CAD build for the part. Positions are in the model's coordinates, mm. A direction names the side the tool comes from. Round coordinates to 2 decimals unless told otherwise and drop trailing zeros. Put each result on its own line as item: value. Start each with the question number.
Item 1: Mould opens along Z. For faces 1 (the flat face through (920.75, 748, -19)), 2 (the flat face through (548, 2136.775, -466)), 3 (the flat face through (83, 1142, -3.175)) say: released by +Z, released by -Z, zero draft, split by the parting line, or undercut.
Item 2: 3-axis set-ups, long thin cutter, end or side, ignore diameter. For faces 4 (the flat face through (914.918, 1053, -454)), 5 (the flat face through (838, 1142, -917.575)), 6 (the flat face through (917.575, 1056, -454)): which of +Z, -Z, +X, -X, +Y, -Y reach the whole face in a straight line?
Item 3: Drill centre lines: line 1 (X direction, y = 477, z = -827.5) (3 decimals); line 2 (Z direction, x = 99, y = 528) (3 decimals); line 3 (Y direction, x = 826, z = -126) (3 decimals). Where is each one in solid material? Low to high. Write a range as from..to.
Item 4: Cut at B-B (z = -780.5). Count the separate pieces of the cut face and the enclosed holes in it, and give its area (3 significant figures).
Item 5: Pin check, flat tips, straight feed: pin 1 Ø10 at (x, z) = (530, -202.5) entering from +Y (3 decimals); pin 2 Ø4 at (y, z) = (661, -553.5) entering from -X (3 decimals); pin 3 Ø2 at (y, z) = (1492, -445.5) entering from +X (3 decimals). Stop position of each tip, or through.
Autodesk Inventor part; units mm, degrees
ref_plane "YZ Plane" through (0, 0, 0) normal (1, 0, 0) x (0, 1, 0)
ref_plane "XZ Plane" through (0, 0, 0) normal (0, 1, 0) x (-1, 0, 0)
ref_plane "XY Plane" through (0, 0, 0) normal (0, 0, 1) x (1, 0, 0)
sketch "Sketch1" plane through (0, 0, 0) normal (0, 1, 0) x (-1, 0, 0)
  line L0 (0, 0) -> (-920.75, 0)
  line L1 (-920.75, 0) -> (-920.75, -920.75)
  line L2 (-920.75, -920.75) -> (0, -920.75)
  line L3 (0, -920.75) -> (0, 0)
  line L4 (-38.1, -38.1) -> (-882.65, -38.1)
  line L5 (-882.65, -38.1) -> (-882.65, -882.65)
  line L6 (-882.65, -882.65) -> (-38.1, -882.65)
  line L7 (-38.1, -882.65) -> (-38.1, -38.1)
  dimension "d0" = 920.75
  dimension "d3" = 920.75
  dimension "d4" = 38.1
  dimension "d5" = 38.1
  dimension "d6" = 38.1
  dimension "d7" = 38.1
extrude "Extrusion1" add sketch "Sketch1" along normal blind 3.175
sketch "Sketch2" plane through (0, 3.175, 0) normal (0, 1, 0) x (1, 0, 0)
  line L0 (0, 0) -> (920.75, 0)
  line L1 (920.75, 0) -> (920.75, 920.75)
  line L2 (920.75, 920.75) -> (0, 920.75)
  line L3 (0, 0) -> (920.75, 0)
  line L4 (920.75, 0) -> (920.75, 920.75)
  line L5 (920.75, 920.75) -> (0, 920.75)
  line L6 (0, 920.75) -> (0, 0)
  line L7 (3.175, 3.175) -> (917.575, 3.175)
  line L8 (917.575, 3.175) -> (917.575, 917.575)
  line L9 (917.575, 917.575) -> (3.175, 917.575)
  line L10 (3.175, 917.575) -> (3.175, 3.175)
  dimension "d10" = 3.175
  dimension "d12" = 3.175
  dimension "d13" = 3.175
  dimension "d14" = 3.175
extrude "Extrusion2" add sketch "Sketch2" along normal blind 34.925
sketch "Sketch3" plane through (0, 38.1, 0) normal (0, 1, 0) x (1, 0, 0)
  line L0 (3.175, 3.175) -> (3.175, 917.575)
  line L1 (917.575, 917.575) -> (917.575, 3.175)
  line L2 (917.575, 3.175) -> (3.175, 3.175)
  line L3 (0, 0) -> (920.75, 0)
  line L4 (920.75, 0) -> (920.75, 920.75)
  line L5 (0, 920.75) -> (0, 0)
  line L6 (0, 0) -> (38.1, 0)
  line L7 (38.1, 3.175) -> (3.175, 3.175)
  line L8 (3.175, 38.1) -> (0, 38.1)
  line L9 (38.1, 0) -> (38.1, 3.175)
  line L10 (920.75, 0) -> (920.75, 38.1)
  line L11 (917.575, 38.1) -> (917.575, 3.175)
  line L12 (882.65, 3.175) -> (882.65, 0)
  line L13 (917.575, 38.1) -> (920.75, 38.1)
  dimension "d17" = 38.1
  dimension "d18" = 38.1
  dimension "d19" = 38.1
  dimension "d20" = 38.1
  dimension "d21" = 38.1
  dimension "d22" = 38.1
extrude "Extrusion3" add sketch "Sketch3" along normal blind 2063.75 contours L2 L9 L3 L5 L8 L0 | L2 L1 L13 L4 L3 L12
sketch "Sketch4" plane through (0, 38.1, 0) normal (0, 1, 0) x (1, 0, 0)
  line L0 (3.175, 38.1) -> (3.175, 917.575)
  line L1 (3.175, 917.575) -> (917.575, 917.575)
  line L2 (917.575, 917.575) -> (917.575, 38.1)
  line L3 (920.75, 38.1) -> (920.75, 920.75)
  line L4 (920.75, 920.75) -> (0, 920.75)
  line L5 (0, 920.75) -> (0, 38.1)
  line L6 (0, 920.75) -> (0, 882.65)
  line L7 (3.175, 882.65) -> (3.175, 917.575)
  line L8 (38.1, 917.575) -> (38.1, 920.75)
  line L9 (0, 882.65) -> (3.175, 882.65)
  line L10 (920.75, 920.75) -> (882.65, 920.75)
  line L11 (882.65, 917.575) -> (917.575, 917.575)
  line L12 (917.575, 882.65) -> (920.75, 882.65)
  line L13 (882.65, 920.75) -> (882.65, 917.575)
  point P0 (0, 0)
  dimension "d25" = 38.1
  dimension "d26" = 38.1
  dimension "d27" = 38.1
  dimension "d28" = 38.1
extrude "Extrusion4" add sketch "Sketch4" along normal blind 2063.75 contours L9 L5 L4 L8 L1 L0 | L13 L4 L3 L12 L2 L1
sketch "Sketch5" plane through (0, 3.175, 0) normal (0, 1, 0) x (1, 0, 0)
  line L0 (3.175, 3.175) -> (917.575, 3.175)
  line L1 (3.175, 3.175) -> (917.575, 3.175)
  line L2 (917.575, 3.175) -> (917.575, 917.575)
  line L3 (917.575, 917.575) -> (3.175, 917.575)
  line L4 (3.175, 917.575) -> (3.175, 3.175)
  line L5 (5.8318, 5.8318) -> (914.9182, 5.8318)
  line L6 (914.9182, 5.8318) -> (914.9182, 914.9182)
  line L7 (914.9182, 914.9182) -> (5.8318, 914.9182)
  line L8 (5.8318, 914.9182) -> (5.8318, 5.8318)
  point P0 (0, 0)
  dimension "d31" = 914.4
  dimension "d33" = 914.4
  dimension "d34" = 2.6568
  dimension "d35" = 2.6568
  dimension "d36" = 909.0863
  dimension "d37" = 909.0863
extrude "Extrusion5" add sketch "Sketch5" along normal blind 2133.6
sketch "Sketch6" plane through (0, 2101.85, 0) normal (0, 1, 0) x (1, 0, 0)
  line L0 (920.75, 0) -> (0, 0)
  line L1 (0, 0) -> (0, 920.75)
  line L2 (0, 920.75) -> (920.75, 920.75)
  line L3 (920.75, 920.75) -> (920.75, 0)
  line L4 (917.575, 3.175) -> (3.175, 3.175)
  line L5 (3.175, 3.175) -> (3.175, 917.575)
  line L6 (3.175, 917.575) -> (917.575, 917.575)
  line L7 (917.575, 917.575) -> (917.575, 3.175)
  point P0 (0, 0)
  dimension "d40" = 920.75
  dimension "d42" = 920.75
  dimension "d43" = 914.4
  dimension "d44" = 914.4
extrude "Extrusion6" add sketch "Sketch6" along normal blind 38.1
sketch "Sketch7" plane through (0, 2136.775, 0) normal (0, 1, 0) x (1, 0, 0)
  line L0 (5.8318, 5.8318) -> (5.8318, 914.9182)
  line L1 (5.8318, 914.9182) -> (914.9182, 914.9182)
  line L2 (914.9182, 914.9182) -> (914.9182, 5.8318)
  line L3 (914.9182, 5.8318) -> (5.8318, 5.8318)
  line L4 (5.8318, 5.8318) -> (914.9182, 5.8318)
  line L5 (914.9182, 5.8318) -> (914.9182, 914.9182)
  line L6 (914.9182, 914.9182) -> (5.8318, 914.9182)
  line L7 (5.8318, 914.9182) -> (5.8318, 5.8318)
  point P0 (0, 0)
  dimension "d47" = 909.0863
  dimension "d49" = 909.0863
extrude "Extrusion7" add sketch "Sketch7" against normal blind 3.175
sketch "Sketch8" plane through (0, 2136.775, 0) normal (0, 1, 0) x (1, 0, 0)
  line L0 (3.175, 3.175) -> (917.575, 3.175)
  line L1 (917.575, 3.175) -> (917.575, 917.575)
  line L2 (917.575, 917.575) -> (3.175, 917.575)
  line L3 (3.175, 917.575) -> (3.175, 3.175)
  line L4 (3.175, 3.175) -> (917.575, 3.175)
  line L5 (917.575, 3.175) -> (917.575, 917.575)
  line L6 (917.575, 917.575) -> (3.175, 917.575)
  line L7 (3.175, 917.575) -> (3.175, 3.175)
  line L8 (38.1, 38.1) -> (882.65, 38.1)
  line L9 (882.65, 38.1) -> (882.65, 882.65)
  line L10 (882.65, 882.65) -> (38.1, 882.65)
  line L11 (38.1, 882.65) -> (38.1, 38.1)
  point P0 (0, 0)
  dimension "d52" = 914.4
  dimension "d54" = 914.4
  dimension "d55" = 34.925
  dimension "d56" = 34.925
  dimension "d57" = 844.55
  dimension "d58" = 844.55
extrude "Extrusion8" add sketch "Sketch8" along normal blind 3.175
sketch "Sketch9" plane through (38.1, 38.1, -3.175) normal (0, 0, 1) x (1, 0, 0)
  line L0 (844.55, 2063.75) -> (0, 2063.75)
  line L1 (0, 0) -> (0, 2063.75)
  line L2 (844.55, 0) -> (0, 0)
  line L3 (844.55, 0) -> (844.55, 2063.75)
  line L4 (63.5, 2000.25) -> (781.05, 2000.25)
  line L5 (781.05, 2000.25) -> (781.05, 1898.65)
  line L6 (781.05, 1898.65) -> (63.5, 1898.65)
  line L7 (63.5, 1898.65) -> (63.5, 2000.25)
  line L8 (63.5, 1797.05) -> (781.05, 1797.05)
  line L9 (781.05, 1797.05) -> (781.05, 266.7)
  line L10 (781.05, 266.7) -> (63.5, 266.7)
  line L11 (63.5, 266.7) -> (63.5, 1797.05)
  line L12 (63.5, 165.1) -> (781.05, 165.1)
  line L13 (781.05, 165.1) -> (781.05, 63.5)
  line L14 (781.05, 63.5) -> (63.5, 63.5)
  line L15 (63.5, 63.5) -> (63.5, 165.1)
  point P0 (-38.1, -38.1)
  dimension "d61" = 63.5
  dimension "d62" = 0
  dimension "d63" = 0
  dimension "d64" = 63.5
  dimension "d65" = 101.6
  dimension "d66" = 63.5
  dimension "d67" = 101.6
  dimension "d68" = 101.6
  dimension "d69" = 101.6
  dimension "d70" = 63.5
  dimension "d71" = 0
  dimension "d72" = 0
extrude "Extrusion9" cut sketch "Sketch9" against normal blind 2.6568 contours L4 L5 L6 L7 | L8 L9 L10 L11 | L12 L13 L14 L15
sketch "Sketch10" plane through (882.65, 38.1, -917.575) normal (0, 0, -1) x (-1, 0, 0)
  line L0 (844.55, 2063.75) -> (0, 2063.75)
  line L1 (0, 0) -> (0, 2063.75)
  line L2 (844.55, 0) -> (0, 0)
  line L3 (844.55, 0) -> (844.55, 2063.75)
  line L4 (63.5, 2000.25) -> (781.05, 2000.25)
  line L5 (781.05, 2000.25) -> (781.05, 1898.65)
  line L6 (781.05, 1898.65) -> (63.5, 1898.65)
  line L7 (63.5, 1898.65) -> (63.5, 2000.25)
  line L8 (63.5, 1797.05) -> (781.05, 1797.05)
  line L9 (781.05, 1797.05) -> (781.05, 266.7)
  line L10 (781.05, 266.7) -> (63.5, 266.7)
  line L11 (63.5, 266.7) -> (63.5, 1797.05)
  line L12 (63.5, 165.1) -> (781.05, 165.1)
  line L13 (781.05, 165.1) -> (781.05, 63.5)
  line L14 (781.05, 63.5) -> (63.5, 63.5)
  line L15 (63.5, 63.5) -> (63.5, 165.1)
  point P0 (882.65, -38.1)
  dimension "d75" = 63.5
  dimension "d76" = 63.5
  dimension "d77" = 63.5
  dimension "d78" = 101.6
  dimension "d79" = 101.6
  dimension "d80" = 0
  dimension "d81" = 0
  dimension "d82" = 101.6
  dimension "d83" = 101.6
  dimension "d84" = 63.5
  dimension "d85" = 0
  dimension "d86" = 0
extrude "Extrusion10" cut sketch "Sketch10" against normal blind 2.6568 contours L4 L5 L6 L7 | L8 L9 L10 L11 | L12 L13 L14 L15
sketch "Sketch11" plane through (917.575, 38.1, -38.1) normal (1, 0, 0) x (0, 0, -1)
  line L0 (844.55, 2063.75) -> (0, 2063.75)
  line L1 (0, 0) -> (0, 2063.75)
  line L2 (844.55, 0) -> (844.55, 2063.75)
  line L3 (63.5, 2000.25) -> (781.05, 2000.25)
  line L4 (781.05, 2000.25) -> (781.05, 1898.65)
  line L5 (781.05, 1898.65) -> (63.5, 1898.65)
  line L6 (63.5, 1898.65) -> (63.5, 2000.25)
  point P0 (-38.1, -38.1)
  dimension "d89" = 63.5
  dimension "d90" = 63.5
  dimension "d91" = 63.5
  dimension "d92" = 101.6
extrude "Extrusion11" cut sketch "Sketch11" against normal blind 2.6568
sketch "Sketch12" plane through (3.175, 38.1, -882.65) normal (-1, 0, 0) x (0, 0, 1)
  line L0 (844.55, 2063.75) -> (0, 2063.75)
  line L1 (0, 0) -> (0, 2063.75)
  line L2 (844.55, 0) -> (844.55, 2063.75)
  line L3 (63.5, 2000.25) -> (781.05, 2000.25)
  line L4 (781.05, 2000.25) -> (781.05, 1898.65)
  line L5 (781.05, 1898.65) -> (63.5, 1898.65)
  line L6 (63.5, 1898.65) -> (63.5, 2000.25)
  point P0 (882.65, -38.1)
  dimension "d95" = 63.5
  dimension "d96" = 63.5
  dimension "d97" = 63.5
  dimension "d98" = 101.6
extrude "Extrusion12" cut sketch "Sketch12" against normal blind 2.6568
sketch "Sketch13" plane through (0, 2136.775, 0) normal (0, 1, 0) x (1, 0, 0)
  line L0 (920.75, 920.75) -> (0, 920.75)
  line L1 (0, 920.75) -> (0, 0)
  line L2 (409.575, 511.175) -> (511.175, 511.175)
  line L3 (511.175, 511.175) -> (511.175, 409.575)
  line L4 (511.175, 409.575) -> (409.575, 409.575)
  line L5 (409.575, 409.575) -> (409.575, 511.175)
  line L6 (0, 0) -> (920.75, 0)
  line L7 (612.775, 511.175) -> (714.375, 511.175)
  line L8 (714.375, 511.175) -> (714.375, 409.575)
  line L9 (714.375, 409.575) -> (612.775, 409.575)
  line L10 (612.775, 409.575) -> (612.775, 511.175)
  line L11 (206.375, 511.175) -> (307.975, 511.175)
  line L12 (307.975, 511.175) -> (307.975, 409.575)
  line L13 (307.975, 409.575) -> (206.375, 409.575)
  line L14 (206.375, 409.575) -> (206.375, 511.175)
  line L15 (409.575, 714.375) -> (511.175, 714.375)
  line L16 (511.175, 714.375) -> (511.175, 612.775)
  line L17 (511.175, 612.775) -> (409.575, 612.775)
  line L18 (409.575, 612.775) -> (409.575, 714.375)
  line L19 (612.775, 714.375) -> (714.375, 714.375)
  line L20 (714.375, 714.375) -> (714.375, 612.775)
  line L21 (714.375, 612.775) -> (612.775, 612.775)
  line L22 (612.775, 612.775) -> (612.775, 714.375)
  line L23 (206.375, 714.375) -> (307.975, 714.375)
  line L24 (307.975, 714.375) -> (307.975, 612.775)
  line L25 (307.975, 612.775) -> (206.375, 612.775)
  line L26 (206.375, 612.775) -> (206.375, 714.375)
  line L27 (409.575, 307.975) -> (511.175, 307.975)
  line L28 (511.175, 307.975) -> (511.175, 206.375)
  line L29 (511.175, 206.375) -> (409.575, 206.375)
  line L30 (409.575, 206.375) -> (409.575, 307.975)
  line L31 (612.775, 307.975) -> (714.375, 307.975)
  line L32 (714.375, 307.975) -> (714.375, 206.375)
  line L33 (714.375, 206.375) -> (612.775, 206.375)
  line L34 (612.775, 206.375) -> (612.775, 307.975)
  line L35 (206.375, 307.975) -> (307.975, 307.975)
  line L36 (307.975, 307.975) -> (307.975, 206.375)
  line L37 (307.975, 206.375) -> (206.375, 206.375)
  line L38 (206.375, 206.375) -> (206.375, 307.975)
  dimension "d150" = 409.575
  dimension "d151" = 101.6
  dimension "d152" = 409.575
  dimension "d153" = 101.6
  dimension "d154" = 101.6
  dimension "d155" = 101.6
  dimension "d156" = 101.6
  dimension "d157" = 101.6
  dimension "d158" = 101.6
  dimension "d159" = 101.6
  dimension "d160" = 101.6
  dimension "d161" = 101.6
  dimension "d162" = 101.6
  dimension "d163" = 101.6
  dimension "d164" = 101.6
  dimension "d165" = 101.6
  dimension "d166" = 101.6
  dimension "d167" = 101.6
  dimension "d168" = 101.6
  dimension "d169" = 101.6
  dimension "d170" = 101.6
  dimension "d171" = 101.6
  dimension "d172" = 101.6
  dimension "d173" = 101.6
  dimension "d174" = 101.6
  dimension "d175" = 101.6
  dimension "d176" = 101.6
  dimension "d177" = 101.6
  dimension "d178" = 101.6
  dimension "d179" = 101.6
  dimension "d180" = 101.6
  dimension "d181" = 101.6
  dimension "d182" = 101.6
  dimension "d183" = 101.6
  dimension "d184" = 101.6
  dimension "d185" = 101.6
extrude "Extrusion13" cut sketch "Sketch13" against normal blind 3.175
properties part number "Cabinet_3x3x7"
Output values:
1. face 1: zero draft
1. face 2: undercut
1. face 3: released by +Z
2. face 4: none
2. face 5: -Z
2. face 6: +X
3. line 1: 3.175..5.832, 914.918..917.575
3. line 2: -917.575..-914.918, -5.832..-3.175
3. line 3: 2133.6..2136.775
4. separate pieces: 3
4. enclosed holes: 0
4. area: 14,600 mm2
5. pin 1: y = 2136.775
5. pin 2: x = 3.175
5. pin 3: x = 917.575
